from build123d import *

# Parameters (mm, degrees)
F1_DEPTH = 64
F3_W     = 15
F3_H     = 60
F4_DEPTH = 25
F5_R     = 3
F5_R_2   = 4
F6_DEPTH = 25


with BuildPart() as f1:
    # F0 (on Front) → F1 (new body)
    with BuildSketch(Plane.XZ):
        with BuildLine():
            Line((-9.5, 17.720389), (-9.5, 0))
            Line((-9.5, 0), (9.5, 0))
            Line((9.5, 0), (9.5, 17.720389))
            ThreePointArc((9.5, 17.720389), (0, 17), (-9.5, 17.720389))
        make_face()
    extrude(amount=-F1_DEPTH)

    # F3 (on offset) → F4 (cut)
    with BuildSketch(Plane.XY.offset(2)):
        with Locations((0, 32)):
            Rectangle(F3_W, F3_H)
    extrude(amount=F4_DEPTH, mode=Mode.SUBTRACT)

    # F5 (on face) → F6 (cut)
    with BuildSketch(Plane.XY.offset(2)):
        with Locations((0, 12)):
            Circle(F5_R)
        with Locations((0, 32)):
            Circle(F5_R)
        with Locations((0, 52)):
            Circle(F5_R_2)
    extrude(amount=-F6_DEPTH, mode=Mode.SUBTRACT)


solid = f1.part
Check sheet for the modelled part. Datum: model origin and axes. Units: mm. A direction names the side the tool comes from. Give positions to 0.01 mm unless a question says otherwise; leave off trailing zeros. Order: outer loops, then holes, each group sorted by start corner. A loop starts at its lowest first (then second) coordinate and runs counter-clockwise, first axis right, second up. Notation, with made-up numbers: M 73,61.5 L 86,61.5 A17 ccw 86,79.5 Z; hole C -6.5,73.5 d3. An arc over 180 degrees is marked long. Answer as CSV lines item,"result". Start each with the question number.
Item 1: Cross-section at B-B on y = 32. Enter the section's corners in (x, z).
Item 2: Mould release check, pull along X, two halves, no side actions. Record for faces 3 (the face through (0, 0, 9)), 4 (the face through (7.5, 32, 10)), 5 (the face through (9.5, 32, 9)): +X half, -X half, draft (parallel to the pull), parting line (faces both ways), or undercut.
Item 3: Gauge pin test, flat ends, axial feed: P1, Ø8, axis at x = 0, y = 32, coming from the +Z side; P2, Ø5, axis at x = 0, y = 52, coming from the -Z side. Record the tip position at first contact, or that the pin passes through.
Item 4: Tool access check on faces 1 (the face through (0, 64, 9)), 2 (the face through (-7.5, 32, 10)). Record the directions out of +Z, -Z, +X, -X, +Y, -Y that give a thin tool (end or side, any length) a straight path to the whole face; none if there is none.
Item 5: Cross-section at A-A on x = 0. Enter the section's corners in (y, z), plus the area to 3 significant figures.
Item 6: Cross-section at D-D on y = 39.5. Enter the section's corners in (x, z), plus the area to 3 significant figures.
Item 7: Cross-section at C-C on z = 9.5. Enter the section's corners in (x, y).
Item 8: Thickness scan on line 1 (Y direction, x = 2, z = 9.75); line 2 (Y direction, x = 0, z = 1.15); line 3 (X direction, y = 47.5, z = 12.25). Record the ranges inside material, lowest first. Write a range as [from, to].
Established:
1,outline,"M -9.5,0 L -3,0 L -3,2 L -7.5,2 L -7.5,17.45 A63 cw -9.5,17.72 Z; M 3,0 L 9.5,0 L 9.5,17.72 A63 cw 7.5,17.45 L 7.5,2 L 3,2 Z"
2,face 3,"draft"
2,face 4,"undercut"
2,face 5,"+X half"
3,P1,"stops at z = 2"
3,P2,"passes through"
4,face 1,"+Z, -Z, +X, -X, +Y"
4,face 2,"+Z"
5,outline,"M 0,0 L 9,0 L 9,2 L 2,2 L 2,17 L 0,17 Z; M 15,0 L 29,0 L 29,2 L 15,2 Z; M 35,0 L 48,0 L 48,2 L 35,2 Z; M 56,0 L 64,0 L 64,17 L 62,17 L 62,2 L 56,2 Z"
5,area,"148 mm^2"
6,outline,"M -9.5,0 L 9.5,0 L 9.5,17.72 A63 cw 7.5,17.45 L 7.5,2 L -7.5,2 L -7.5,17.45 A63 cw -9.5,17.72 Z"
6,area,"100 mm^2"
7,outline,"M -9.5,0 L 9.5,0 L 9.5,64 L -9.5,64 Z; hole M -7.5,2 L 7.5,2 L 7.5,62 L -7.5,62 Z"
8,line 1,"y = [0, 2], [62, 64]"
8,line 2,"y = [0, 9], [15, 29], [35, 48], [56, 64]"
8,line 3,"x = [-9.5, -7.5], [7.5, 9.5]"
